Design review of the part built by this model. Coordinates are the model's own, in mm. Face numbers are marked on the shaded views. A direction names the side the tool comes from. Round coordinates to 2 decimals unless told otherwise and drop trailing zeros. Order: outer loops, then holes, each group sorted by start corner. A loop starts at its lowest first (then second) coordinate and runs counter-clockwise, first axis right, second up. Notation, with made-up numbers: M 13.25,81 L 66.25,81 A34 ccw 66.25,114 Z; hole C 79,-10.75 d8. An arc over 180 degrees is marked long. Write each question's results on one line, items separated by ' | '. Start each with the question number.
Item 1: The part is to be moulded in two halves that separate along Y. For the marked faces 3, 4, 5 and 6, say which applies: +Y half, -Y half, draft (parallel to the pull), parting line (faces both ways), or undercut.
Item 2: Take a section at B-B, the plane z = 0. Write out the cut boundary in (x, y).
Item 3: Take a section at A-A, the plane x = 0. Write out the cut boundary in (y, z).
Item 4: Take a section at D-D, the plane y = -2. Write out the cut boundary in (x, z) (1 decimal), plus the area to 3 significant figures.
Item 5: Wall thickness on line 1 (Y direction, x = -1.75, z = 0.5); line 2 (Y direction, x = -0.25, z = 2); line 3 (Z direction, x = -1.5, y = -4.95): over which ranges is each line inside the solid? List them lowest first. Write a range as [from, to].
Item 6: Machinability: for the marked faces 1 and 2, which of the approach directions +Z, -Z, +X, -X, +Y, -Y give a long, thin tool a straight path to every point of the face, cutting with its end or side? Answer none if there is none.
Item 7: Take a section at C-C, the plane y = -2.7. Write out the cut boundary in (x, z), plus the area to 3 significant figures.
```python
from build123d import *

# Parameters (mm, degrees)
SKETCH3_R           = 2.1209
BOSS_EXTRUDE1_DEPTH = 7.5692
CUT_EXTRUDE1_START  = -11.811
SKETCH5_R           = 2.1209
CUT_EXTRUDE1_DEPTH  = 8.636
FILLET1_R           = 0.254


with BuildPart() as part:
    # Sketch2 → Revolve1 (revolve)
    with BuildSketch(Plane.XY, mode=Mode.PRIVATE) as revolve1_sk:
        with BuildLine():
            Line((1.5875, -1.397), (1.5875, -10.0584))
            Line((1.5875, -10.0584), (0, -10.0584))
            Line((0, -10.0584), (0, 0))
            Line((0, 0), (2.783660204, 0))
            ThreePointArc((2.783660204, 0), (3.10032913, -0.242988613), (2.947580102, -0.611757387))
            Line((2.947580102, -0.611757387), (1.5875, -1.397))
        make_face()
    revolve(revolve1_sk.sketch.rotate(Axis((0, 94.608881441, 0), (0, -1, 0)), 90), axis=Axis((0, 94.608881441, 0), (0, -1, 0)))

    # Sketch3 → Boss-Extrude1 (add)
    with BuildSketch(Plane.XZ.offset(10.0584)):
        with Locations(Location((0, 0, 0), (0, 0, 270))):
            Circle(SKETCH3_R)
    extrude(amount=-BOSS_EXTRUDE1_DEPTH)

    # Sketch5 → Cut-Extrude1 (cut)
    with BuildSketch(Plane(origin=(0, -2.4892, 0), x_dir=(1, 0, 0), z_dir=(0, 1, 0)).offset(CUT_EXTRUDE1_START)):
        with Locations(Location((0, 0, 0), (0, 0, 90))):
            Circle(SKETCH5_R)
    extrude(amount=CUT_EXTRUDE1_DEPTH, mode=Mode.SUBTRACT)

    # Fillet1
    fillet1_edges = [part.edges().sort_by_distance(p)[0] for p in [
        (0, -5.6642, 2.1209),
    ]]
    fillet(fillet1_edges, radius=FILLET1_R)


solid = part.part
```
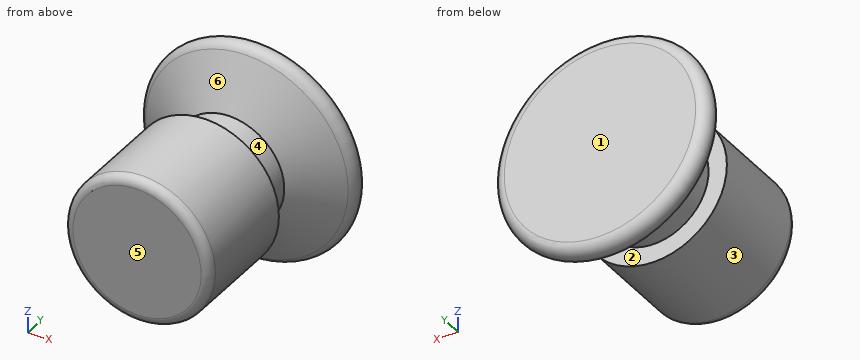
Results list:
1) face 3: draft | face 4: undercut | face 5: -Y half | face 6: undercut
2) outline: M -2.95,-0.61 L -1.59,-1.4 L -1.59,-2.49 L -2.12,-2.49 L -2.12,-5.41 A0.25 ccw -1.87,-5.66 L 1.87,-5.66 A0.25 ccw 2.12,-5.41 L 2.12,-2.49 L 1.59,-2.49 L 1.59,-1.4 L 2.95,-0.61 A0.33 ccw 2.78,0 L -2.78,0 A0.33 ccw Z
3) outline: M -5.66,-1.87 A0.25 ccw -5.41,-2.12 L -2.49,-2.12 L -2.49,-1.59 L -1.4,-1.59 L -0.61,-2.95 A0.33 ccw 0,-2.78 L 0,2.78 A0.33 ccw -0.61,2.95 L -1.4,1.59 L -2.49,1.59 L -2.49,2.12 L -5.41,2.12 A0.25 ccw -5.66,1.87 Z
4) outline: C 0,0 d3.2 | area: 7.92 mm²
5) line 1: [-5.66, -2.49], [-1.26, 0] | line 2: [-5.62, -2.49], [-1.15, 0] | line 3: [-1.5, 1.5]
6) face 1: +Z, -Z, +X, -X, +Y | face 2: none
7) outline: C 0,0 d4.24 | area: 14.1 mm²
